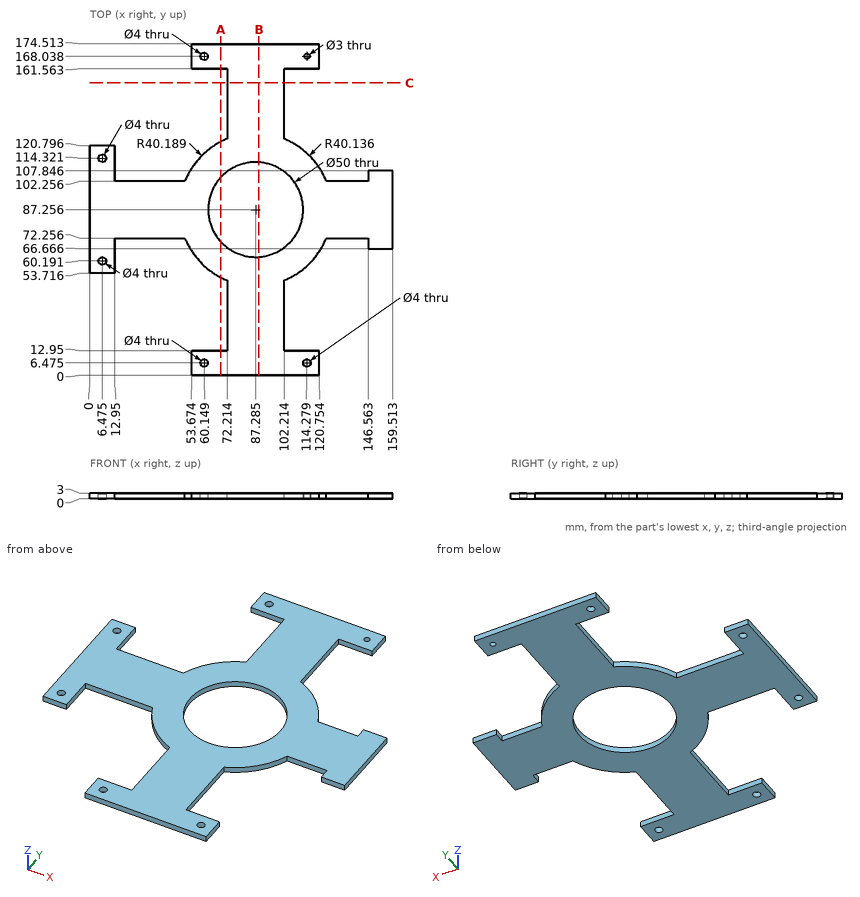
Check sheet for the drawn part. Datum: minimum x, y, z corner. Units: mm. Give positions to 0.01 mm unless a question says otherwise; leave off trailing zeros. Write each loop counter-clockwise with the first axis right and the second up, starting at its lowest first coordinate (ties: lowest second). Pieces come first, ordered by that corner, then holes. Notation, with made-up numbers: (11, -17) -> (25, -17) arc R14 cw to (25, 0) -> close; hole circle Ø3 at (44.5, -37.5). An arc over 180 degrees is marked (long way). Use one line per item in the form item = value. Start each with the question number.
1. Section check B-B (x = 89). Record the cut outline in (y, z) (1 decimal).
2. Go/stop test with flat-tipped pins: P1, Ø1, axis at y = 24.5, z = 0.5, coming from the -X side; P2, Ø1, axis at x = 23, z = 1.5, coming from the -Y side; P3, Ø0.9, axis at y = 36, z = 1, coming from the +X side. Record where each tip stops, or that it passes through.
3. Section check A-A (x = 69). Count the separate pieces of the cut face and the enclosed holes in it, and give its area (3 significant figures).
4. Section check C-C (y = 154). Record the cut outline in (x, z) (1 decimal).
5. Thickness scan on line 1 along X through (y, z) = (154.5, 2.3) (1 decimal); line 2 along X through (y, z) = (93, 1.75) (1 decimal); line 3 along X through (y, z) = (74, 1.95) (1 decimal). Record the ranges inside material, lowest first. Write a range as from..to.
Conclusion:
q1.outline = (0, 0) -> (62.3, 0) -> (62.3, 3) -> (0, 3) -> close; (112.2, 0) -> (174.5, 0) -> (174.5, 3) -> (112.2, 3) -> close
q2.P1 = 72.21
q2.P2 = 72.26
q2.P3 = 102.21
q3.separate_pieces = 4
q3.enclosed_holes = 0
q3.area = 190 mm²
q4.outline = (72.2, 0) -> (102.2, 0) -> (102.2, 3) -> (72.2, 3) -> close
q5.line_1 = 72.2..102.2
q5.line_2 = 0..63, 111.6..159.5
q5.line_3 = 0..66.1, 108.5..159.5
